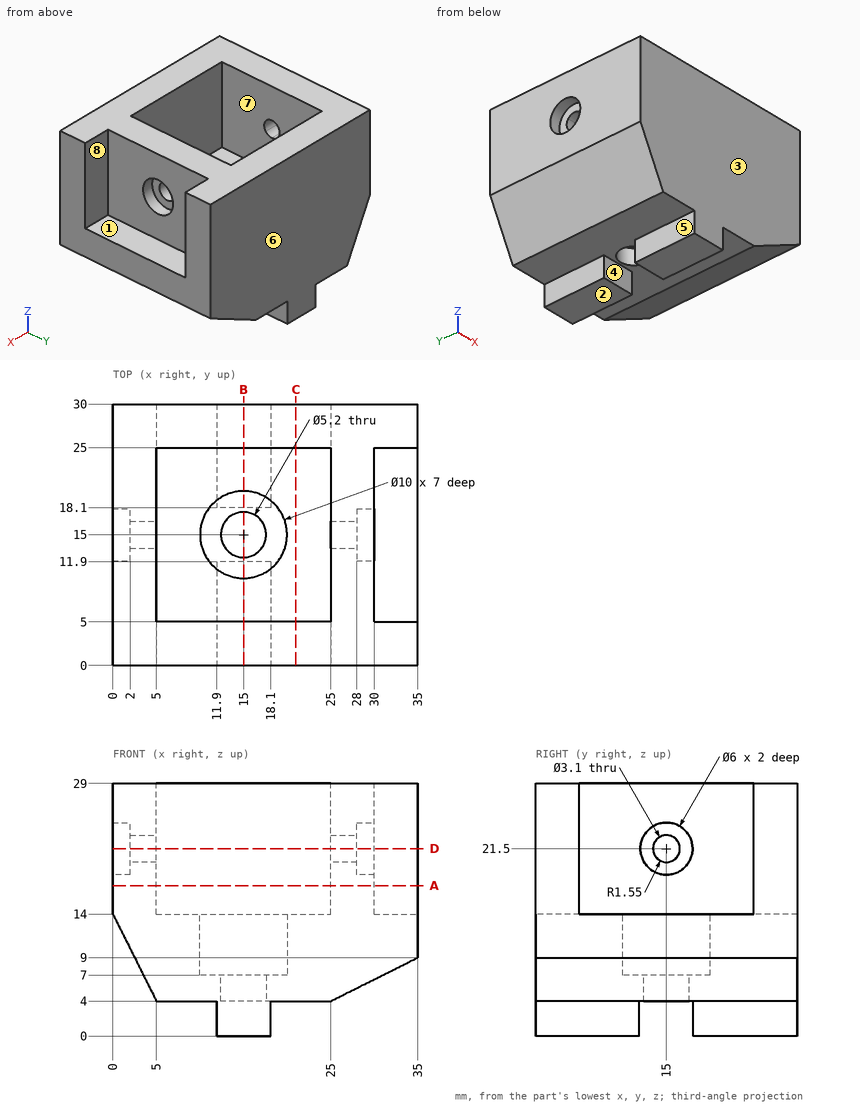
Here's the drawing with two shaded views (mm, measured from the low corner). I have some questions. A direction names the side the tool comes from. Round coordinates to 2 decimals unless told otherwise and drop trailing zeros. Loops run counter-clockwise (first coordinate to the right, second up) from the corner with the lowest first, then second, coordinate; pieces in that order, holes last.
Item 1: Suppose I cut it at B-B, the plane x = 15. Write out the boundary of the cut face in (y, z).
Item 2: Suppose I cut it at A-A, the plane z = 17.25. Write out the boundary of the cut face in (x, y), then the cut area to 3 significant figures.
Item 3: Which directions (+Z, -Z, +X, -X, +Y, -Y) give clear straight access to the entire face, cutting with the end or side of a thin tool? Please do the marked faces 5, 6, 7 and 8.
Item 4: Suppose I cut it at D-D, the plane z = 21.5. Write out the boundary of the cut face in (x, y), then the cut area to 3 significant figures.
Item 5: Suppose I cut it at C-C, the plane x = 21. Write out the boundary of the cut face in (y, z), then the cut area to 3 significant figures.
Item 6: Please list where these lines run through material, in increasing order: L1, parallel to Y at x = 15, z = 5.05; L2, parallel to Y at x = 15, z = 8.5; L3, parallel to X at y = 9, z = 21.75.
Item 7: If we mould it in two halves opening along Y, with no side actions, what happens to the marked faces 1, 2, 3 and 4? For each: +Y half, -Y half, draft (parallel to the pull), parting line (faces both ways), or undercut.
Item 8: Will these pins go through, and if not, where does the flat tip stop? pin 1 Ø12 at (y, z) = (14.5, 6.5) entering from -X; pin 2 Ø2 at (y, z) = (5, 2.5) entering from +X; pin 3 Ø1.8 at (y, z) = (14.5, 23) entering from +X.
Reported:
1. outline: (0, 0) - (11.9, 0) - (11.9, 4) - (12.4, 4) - (12.4, 7) - (10, 7) - (10, 14) - (5, 14) - (5, 29) - (0, 29) - close; (17.6, 4) - (18.1, 4) - (18.1, 0) - (30, 0) - (30, 29) - (25, 29) - (25, 14) - (20, 14) - (20, 7) - (17.6, 7) - close
2. outline: (0, 0) - (35, 0) - (35, 5) - (30, 5) - (30, 25) - (35, 25) - (35, 30) - (0, 30) - close; hole (5, 5) - (25, 5) - (25, 25) - (5, 25) - close
2. area: 550 mm2
3. face 5: -Z, -X, +Y, -Y
3. face 6: +Z, -Z, +X, -X, +Y
3. face 7: +Z
3. face 8: +Z, +X
4. outline: (0, 0) - (35, 0) - (35, 5) - (30, 5) - (30, 12) - (28, 12) - (28, 13.45) - (25, 13.45) - (25, 5) - (5, 5) - (5, 13.45) - (2, 13.45) - (2, 12) - (0, 12) - close; (0, 18) - (2, 18) - (2, 16.55) - (5, 16.55) - (5, 25) - (25, 25) - (25, 16.55) - (28, 16.55) - (28, 18) - (30, 18) - (30, 25) - (35, 25) - (35, 30) - (0, 30) - close
4. area: 507 mm2
5. outline: (0, 4) - (30, 4) - (30, 29) - (25, 29) - (25, 14) - (5, 14) - (5, 29) - (0, 29) - close
5. area: 450 mm2
6. L1: y = 0 to 12.4, 17.6 to 30
6. L2: y = 0 to 10, 20 to 30
6. L3: x = 0 to 5, 25 to 30
7. face 1: undercut
7. face 2: draft
7. face 3: -Y half
7. face 4: undercut
8. pin 1: stops at x = 0.75
8. pin 2: stops at x = 18.1
8. pin 3: stops at x = 28
